Geometry check sheet. Reference: drawing and pictorial views, mm from the part's lowest x, y, z. A direction names the side the tool comes from. Give positions to 0.01 mm unless a question says otherwise; leave off trailing zeros. Order: outer loops, then holes, each group sorted by start corner. A loop starts at its lowest first (then second) coordinate and runs counter-clockwise, first axis right, second up. Notation, with made-up numbers: M 34.5,7 L 56.5,7 A22 ccw 56.5,26 Z; hole C 65.25,-7.5 d10. An arc over 180 degrees is marked long. Answer as CSV lines item,"result". Start each with the question number.
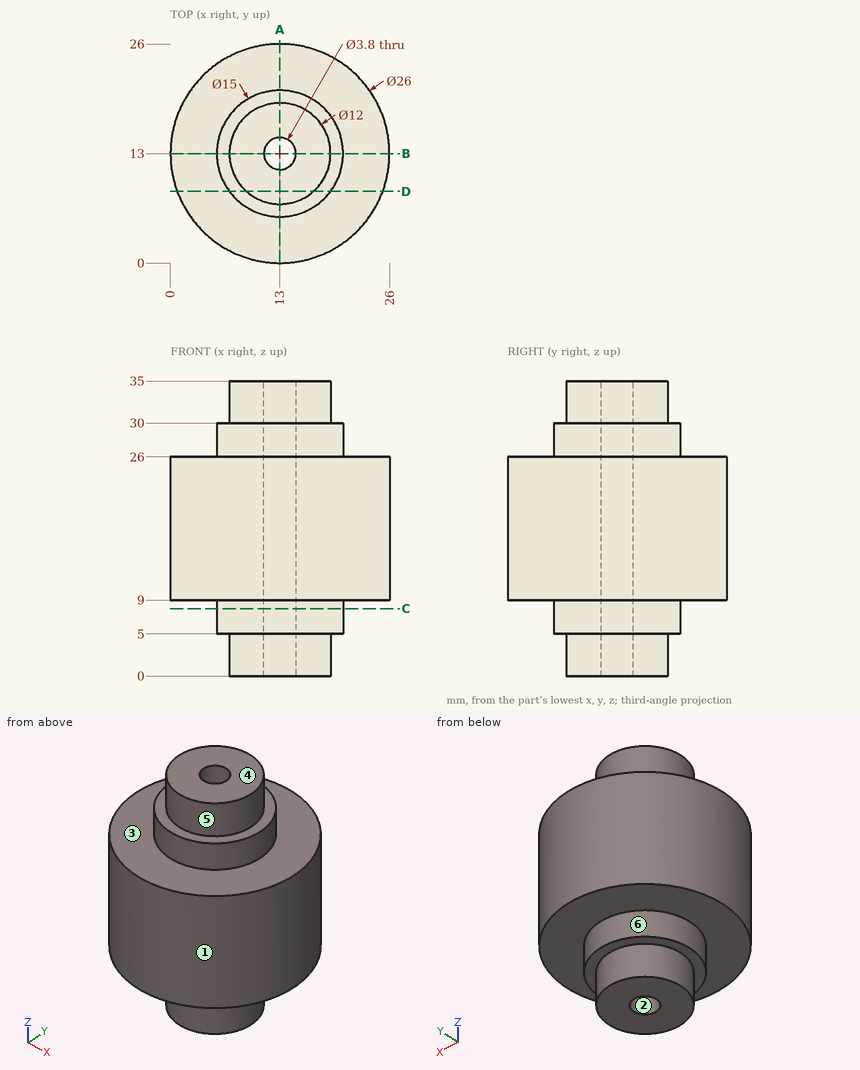
Item 1: Section check D-D on y = 8.5. Record the boundary of the cut face in (x, z).
Item 2: Section check C-C on z = 8. Record the boundary of the cut face in (x, y).
Item 3: Section check A-A on x = 13. Record the boundary of the cut face in (y, z), then the cut area to 3 significant figures.
Item 4: Depth check by flat-ended pin: pin 1 Ø4 at (x, y) = (4.5, 13.5) entering from -Z; pin 2 Ø5 at (y, z) = (22, 19.5) entering from -X; pin 3 Ø3 at (x, z) = (20.5, 25) entering from -Y; pin 4 Ø3 at (x, y) = (13, 13) entering from +Z. Enter the tip coordinate at first touch or a pass-through.
Item 5: Access from +Z, -Z, +X, -X, +Y, -Y to the whole of each face (thin tool, end or side, straight path). Record for the marked faces 4, 5 and 6.
Item 6: Draft check along Y on the marked faces 1, 2 and 3. Enter one of: pulls with the +Y half, pulls with the -Y half, needs draft (parallel to the pull), parting line crosses it, or undercut.
Item 7: Scan lines: line 1 along Y through (x, z) = (13, 17.5); line 2 along Z through (x, y) = (5.75, 19.5); line 3 along Y through (x, z) = (13.75, 28). Record each from-to range of solid material in increasing order.
Numbers:
1,outline,"M 0.8,9 L 7,9 L 7,5 L 9.03,5 L 9.03,0 L 16.97,0 L 16.97,5 L 19,5 L 19,9 L 25.2,9 L 25.2,26 L 19,26 L 19,30 L 16.97,30 L 16.97,35 L 9.03,35 L 9.03,30 L 7,30 L 7,26 L 0.8,26 Z"
2,outline,"C 13,13 d15; hole C 13,13 d3.8"
3,outline,"M 0,9 L 5.5,9 L 5.5,5 L 7,5 L 7,0 L 11.1,0 L 11.1,35 L 7,35 L 7,30 L 5.5,30 L 5.5,26 L 0,26 Z; M 14.9,0 L 19,0 L 19,5 L 20.5,5 L 20.5,9 L 26,9 L 26,26 L 20.5,26 L 20.5,30 L 19,30 L 19,35 L 14.9,35 Z"
3,area,"549 mm2"
4,pin 1,"z = 5"
4,pin 2,"x = 1.74"
4,pin 3,"y = 1.47"
4,pin 4,"through"
5,face 4,"+Z, +X, -X, +Y, -Y"
5,face 5,"+Z"
5,face 6,"-Z"
6,face 1,"parting line crosses it"
6,face 2,"undercut"
6,face 3,"needs draft"
7,line 1,"0 to 11.1, 14.9 to 26"
7,line 2,"9 to 26"
7,line 3,"5.54 to 11.25, 14.75 to 20.46"
